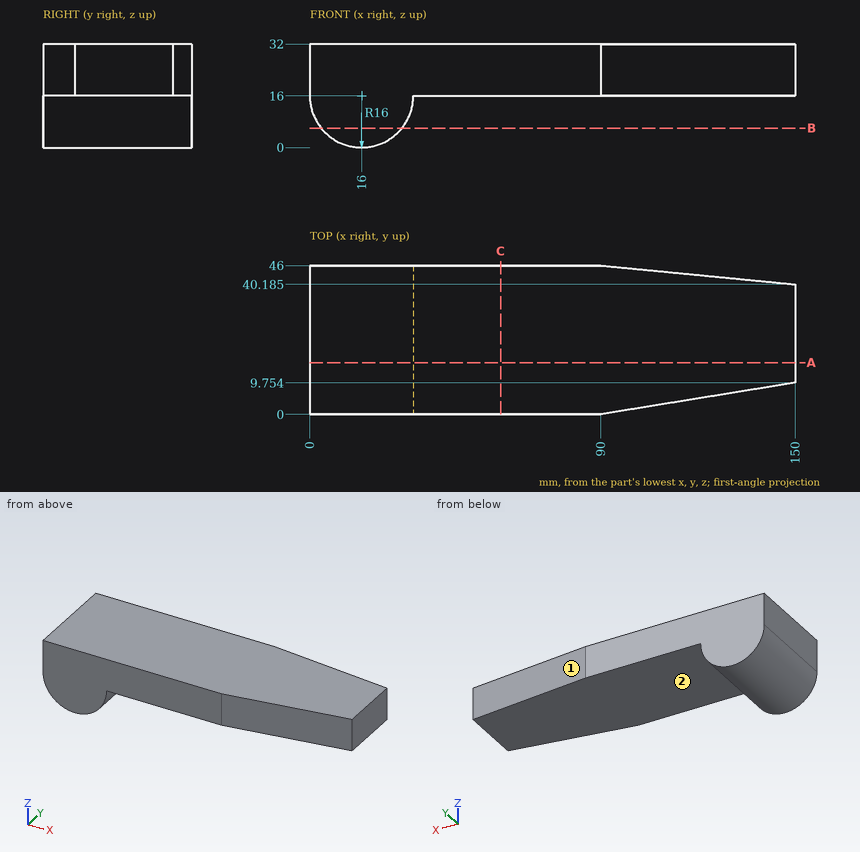
Geometry: see drawing. Coordinates: mm, zero at the bounding-box minimum. A direction names the side the tool comes from. Give positions to 0.01 mm unless a question says otherwise; leave off trailing zeros. Order: outer loops, then holes, each group sorted by start corner. A loop starts at its lowest first (then second) coordinate and runs counter-clockwise, first axis right, second up. Notation, with made-up numbers: (72, 33.5) - (84, 33.5) arc R21 cw to (84, 41.5) - close; hole circle Ø2 at (87.25, 36). An arc over 180 degrees is marked (long way). Use CSV: the item, a comma, the result in double quotes.
1. Section query C-C (x = 59). Output: boundary loops of the cut face in (y, z), plus the area to 3 significant figures.
Answers below:
outline,"(0, 16) - (46, 16) - (46, 32) - (0, 32) - close"
area,"736 mm2"
2. Access query for the marked faces 1 and 2. Directions: +Z, -Z, +X, -X, +Y, -Y. A direction counts if a zero-diameter tool reaches every point of the face in a straight line with its end or side. Return the directions, or none.
Answers below:
face 1,"+Z, -Z, +X, +Y"
face 2,"-Z, +X, +Y, -Y"
3. Material intervals for line 1 along Z through (x, y) = (137.5, 21); line 2 along X through (y, z) = (12.5, 15); line 3 along Z through (x, y) = (28, 13) (1 decimal), sorted ascending. Write a range as from..to.
Answers below:
line 1,"16..32"
line 2,"0.03..31.97"
line 3,"5.4..32"
4. Contact query for flat-ended pins moving along their axis: pin 1 (1.5 mm diameter, centred on x = 99.5, y = 12, fed in from -Z); pin 2 (5 mm diameter, centred on x = 119.5, z = 23.5, fed in from +Y). Output: stop coordinate, or through.
Answers below:
pin 1,"z = 16"
pin 2,"y = 43.38"
5. Section query A-A (y = 16). Output: boundary loops of the cut face in (x, z), plus the area to 3 significant figures.
Answers below:
outline,"(0, 16) arc R16 ccw to (32, 16) - (150, 16) - (150, 32) - (0, 32) - close"
area,"2,800 mm2"
6. Section query B-B (z = 6). Output: boundary loops of the cut face in (x, y).
Answers below:
outline,"(3.51, 0) - (28.49, 0) - (28.49, 46) - (3.51, 46) - close"
